Geometry: final body of the model. Coordinates: model frame, mm. A direction names the side the tool comes from. Give positions to 0.01 mm unless a question says otherwise; leave off trailing zeros. Order: outer loops, then holes, each group sorted by start corner. A loop starts at its lowest first (then second) coordinate and runs counter-clockwise, first axis right, second up. Notation, with made-up numbers: M 65.25,-33 L 104.25,-33 A20 cw 104.25,-21 Z; hole C 88,11 d11. An arc over 180 degrees is marked long. Write item = value, one per line. Start each with the question number.
Autodesk Inventor part; units mm, degrees
ref_plane "Arbeitsebene1" through (6, 0, 0) normal (1, 0, 0) x (0, 1, 0)
ref_plane "XZ Plane" through (0, 0, 0) normal (0, 1, 0) x (-1, 0, 0)
ref_plane "XY Plane" through (0, 0, 0) normal (0, 0, 1) x (1, 0, 0)
sketch "Skizze1" plane through (0, 0, 0) normal (0, 0, 1) x (1, 0, 0)
  line L0 (-8.4, 0) -> (8.4, 0)
  line L1 (0, -8.4) -> (0, 8.4)
  circle A0 centre (0, 0) radius 6
  dimension "d0" = 12
extrude "Extrusion1" add sketch "Skizze1" along normal blind 120
sketch "Skizze2" plane through (0, 0, 120) normal (0, 0, 1) x (1, 0, 0)
  circle A0 centre (0, 0) radius 6
  circle A1 centre (0, 0) radius 3
  dimension "d3" = 6
extrude "Extrusion2" cut sketch "Skizze2" against normal blind 7.5
sketch "Skizze3" plane through (0, 0, 0) normal (0, 0, -1) x (-1, 0, 0)
  circle A0 centre (0, 0) radius 6
  circle A1 centre (0, 0) radius 3
  circle A2 centre (0, 0) radius 3
extrude "Extrusion3" cut sketch "Skizze3" against normal blind 7.5
sketch "Skizze4" plane through (0, 0, 0) normal (0, 0, -1) x (-1, 0, 0)
  circle A0 centre (0, 0) radius 3
hole "Bohrung1" at (0, 0, 0) direction (0, 0, 1) diameter 4.134 depth 14.2 tip angle 118
sketch "Skizze5" plane through (0, 0, 120) normal (0, 0, 1) x (1, 0, 0)
  point P0 (0, 0)
  point P1 (0, 0)
hole "Bohrung2" at (0, 0, 120) direction (0, 0, -1) diameter 4.134 depth 14.2 tip angle 118
ref_plane "Arbeitsebene1" through (6, 0, 0) normal (1, 0, 0) x (0, 1, 0)
sketch "Skizze7" plane through (6, 0, 0) normal (1, 0, 0) x (0, 1, 0)
  line L0 (-6, 112.5) -> (6, 112.5)
  line L1 (-6, 7.5) -> (-6, 112.5)
  line L2 (6, 7.5) -> (6, 112.5)
  line L3 (-6, 112.5) -> (6, 112.5)
  line L4 (6, 112.5) -> (6, 90.5)
  line L5 (6, 90.5) -> (-6, 90.5)
  line L6 (-6, 90.5) -> (-6, 112.5)
  arc A0 (-6, 90.5) -> (6, 90.5) centre (0, 90.5) ccw
  line L7 (-8.4, 0) -> (8.4, 0)
  line L8 (0, -24) -> (0, 144)
  point P0 (0, 0)
  dimension "d22" = 22
extrude "Extrusion4" cut sketch "Skizze7" against normal blind 3
sketch "Skizze8" plane through (3, 0, 0) normal (1, 0, 0) x (0, 0, -1)
  line L0 (0, -8.4) -> (0, 8.4)
  line L1 (24, 0) -> (-144, 0)
  line L2 (-109, -2.5) -> (-99, -2.5) construction
  line L3 (-87.5, -5.1962) -> (-112.5, -5.1962)
  line L4 (-99, 2.5) -> (-109, 2.5) construction
  line L5 (-109, -2.5) -> (-99, -2.5) construction
  line L6 (-109, -1.25) -> (-99, -1.25)
  line L7 (-99, -3.75) -> (-109, -3.75)
  arc A0 (-109, -1.25) -> (-109, -3.75) centre (-109, -2.5) ccw
  arc A1 (-99, -3.75) -> (-99, -1.25) centre (-99, -2.5) ccw
  line L8 (-109, 2.5) -> (-99, 2.5) construction
  line L9 (-109, 3.75) -> (-99, 3.75)
  line L10 (-99, 1.25) -> (-109, 1.25)
  arc A2 (-109, 3.75) -> (-109, 1.25) centre (-109, 2.5) ccw
  arc A3 (-99, 1.25) -> (-99, 3.75) centre (-99, 2.5) ccw
  line L11 (-112.5, 0) -> (-112.5, 5.1962)
  line L12 (-112.5, -5.1962) -> (-112.5, 0)
  point P0 (0, 0)
  point P1 (-104, -2.5)
  point P2 (-104, 2.5)
  dimension "d25" = 5
  dimension "d26" = 2.5
  dimension "d27" = 2.5
  dimension "d28" = 3.5
  dimension "d29" = 3.5
  dimension "d30" = 10
  dimension "d31" = 10
extrude "Extrusion5" cut sketch "Skizze8" against normal blind 1.3
sketch "Skizze9" plane through (3, 0, 0) normal (1, 0, 0) x (0, 0, -1)
  line L0 (24, 0) -> (-144, 0)
  line L1 (0, -8.4) -> (0, 8.4)
  line L2 (-112.5, -5.1962) -> (-112.5, 0)
  point P0 (0, 0)
  point P1 (-94.5, 0)
  dimension "d34" = 18
hole "Bohrung3" at (3, 0, 94.5) direction (-1, 0, 0) diameter 3.242 depth 11.8 tip angle 118
sketch "Skizze10" plane through (3, 0, 0) normal (1, 0, 0) x (0, 0, -1)
  line L0 (24, 0) -> (-144, 0)
  line L1 (0, -8.4) -> (0, 8.4)
  circle A0 centre (-94.5, 0) radius 1.621
  point P0 (0, 0)
  point P1 (-87.5, 0)
  dimension "d42" = 7
hole "Bohrung4" at (3, 0, 87.5) direction (-1, 0, 0) diameter 3 end through all
equation "\"d27\" = d26"
equation "\"d29\" = d28"
equation "\"d31\" = d30"
properties part number "24_0497_004"
1) Pin query (flat end, axial travel): pin 1 Ø3 at (y, z) = (-0.5, 100) entering from -X; pin 2 Ø1 at (x, z) = (2.5, 102.5) entering from +Y; pin 3 Ø3 at (y, z) = (2.5, 102) entering from +X; pin 4 Ø1.4 at (x, z) = (2, 103) entering from -Y. Return the tip coordinate at first contact, or that it passes through.
2) Cut plane D-D (z = 48). Return loops of the section in (x, y), plus the area to 3 significant figures.
3) Access query for faces 1 (the cylindrical face through (1.26, 1.64, 112.8)), 2 (the flat face through (1.7, -2, 104)), 3 (the cylindrical face through (1.26, -1.64, 7.2)). Directions: +Z, -Z, +X, -X, +Y, -Y. A direction counts if a zero-diameter tool reaches every point of the face in a straight line with its end or side. Return the directions, or none.
4) Cut plane C-C (x = -4.75). Return loops of the section in (y, z).
5) Cut plane B-B (z = 9). Return loops of the section in (x, y).
6) Cut plane A-A (z = 94.5). Return loops of the section in (x, y).
7) Draft query along Y for faces 4 (the cylindrical face through (-3, 0, 116)), 5 (the cylindrical face through (-1.563, -0.487, 92.954)), 6 (the flat face through (3, -1, 7.5)). Return one class per face: pulls with the +Y half, pulls with the -Y half, needs draft (parallel to the pull), parting line crosses it, or undercut.
8) Ray query, L1, parallel to Y at x = 0, z = 9.5; L2, parallel to Y at x = 0, z = 115; L3, parallel to Z at x = -1, y = 0. Return the intervals inside material, ascending.
Reply:
q1.pin_1 = -6
q1.pin_2 = 5.66
q1.pin_3 = 3
q1.pin_4 = -5.86
q2.outline = C 0,0 d12
q2.area = 113 mm²
q3.face_1 = +Z
q3.face_2 = +X
q3.face_3 = -Z
q4.outline = M -3.67,7.5 L 3.67,7.5 L 3.67,112.5 L -3.67,112.5 Z; hole C 0,94.5 d3.24; hole C 0,87.5 d3
q5.outline = C 0,0 d12; hole C 0,0 d4.13
q6.outline = M -5.78,-1.62 A6 ccw 3,-5.2 L 3,-1.62 Z; M -5.78,1.62 L 3,1.62 L 3,5.2 A6 ccw Z
q7.face_4 = parting line crosses it
q7.face_5 = undercut
q7.face_6 = needs draft
q8.L1 = -6 to -2.07, 2.07 to 6
q8.L2 = -3 to -2.07, 2.07 to 3
q8.L3 = 14.84 to 86, 89 to 92.88, 96.12 to 105.16
